Design review of the part built by this model. Coordinates are the model's own, in mm. A direction names the side the tool comes from. Give positions to 0.01 mm unless a question says otherwise; leave off trailing zeros. Order: outer loops, then holes, each group sorted by start corner. A loop starts at its lowest first (then second) coordinate and runs counter-clockwise, first axis right, second up. Notation, with made-up numbers: (-12, 69.25) -> (27, 69.25) arc R18 ccw to (27, 102.25) -> close; hole circle Ø2 at (46.5, -18). An arc over 180 degrees is marked (long way). Return JSON: item names as keys, results as strings.
```python
from build123d import *

# Parameters (mm, degrees)
SKETCH1_R           = 3.75
BOSS_EXTRUDE1_DEPTH = 3.175
SKETCH2_R           = 1.984375
CUT_EXTRUDE1_DEPTH  = 4.175
SKETCH3_W           = 57.15
SKETCH3_H           = 3.175
BOSS_EXTRUDE2_DEPTH = 19.05
SKETCH4_W           = 2.38125
SKETCH4_H           = 2.032
BOSS_EXTRUDE3_DEPTH = 4.7625
SKETCH5_R           = 2.0955
CUT_EXTRUDE2_DEPTH  = 4.175
CHAMFER1_SIZE       = 0.79375
CHAMFER3_SIZE       = 1.5875
FILLET1_R           = 3.175


with BuildPart() as part:
    # Sketch1 → Boss-Extrude1 (new body)
    with BuildSketch(Plane(origin=(0, 0, 0), x_dir=(0, 0, -1), z_dir=(1, 0, 0))):
        with BuildLine():
            Line((-28.575, 0), (28.575, 0))
            Line((28.575, 0), (28.575, 3.175))
            Line((28.575, 3.175), (20.6375, 3.175))
            Line((20.6375, 3.175), (11.1125, 12.7))
            ThreePointArc((11.1125, 12.7), (0, 23.8125), (-11.1125, 12.7))
            Line((-11.1125, 12.7), (-20.6375, 3.175))
            Line((-20.6375, 3.175), (-28.575, 3.175))
            Line((-28.575, 3.175), (-28.575, 0))
        make_face()
        with Locations((0, 12.7)):
            Circle(SKETCH1_R, mode=Mode.SUBTRACT)
    extrude(amount=-BOSS_EXTRUDE1_DEPTH)

    # Sketch2 → Cut-Extrude1 (cut, through all)
    with BuildSketch(Plane(origin=(0, 0, 0), x_dir=(0, 0, -1), z_dir=(1, 0, 0))):
        with Locations((0, 19.812)):
            Circle(SKETCH2_R)
    extrude(amount=-CUT_EXTRUDE1_DEPTH, mode=Mode.SUBTRACT)

    # Sketch3 → Boss-Extrude2 (add)
    with BuildSketch(Plane.ZY.offset(3.175)):
        with Locations((0, 1.5875)):
            Rectangle(SKETCH3_W, SKETCH3_H)
    extrude(amount=BOSS_EXTRUDE2_DEPTH)

    # Sketch4 → Boss-Extrude3 (add)
    with BuildSketch(Plane.ZY.offset(3.175)):
        with Locations((9.128125, 4.191)):
            Rectangle(SKETCH4_W, SKETCH4_H)
    extrude(amount=BOSS_EXTRUDE3_DEPTH)

    # Sketch5 → Cut-Extrude2 (cut, through all)
    with BuildSketch(Plane(origin=(0, 3.175, 0), x_dir=(1, 0, 0), z_dir=(0, 1, 0))):
        with Locations((-11.1125, -19.05)):
            Circle(SKETCH5_R)
        with Locations((-11.1125, 19.05)):
            Circle(SKETCH5_R)
    extrude(amount=-CUT_EXTRUDE2_DEPTH, mode=Mode.SUBTRACT)

    # Chamfer1
    chamfer1_edges = [part.edges().sort_by_distance(p)[0] for p in [
        (-13.208, 3.175, 19.05),
        (-13.208, 3.175, -19.05),
    ]]
    chamfer(chamfer1_edges, length=CHAMFER1_SIZE)

    # Chamfer3
    chamfer3_edges = [part.edges().sort_by_distance(p)[0] for p in [
        (-3.175, 3.175, 15.478125),
        (-3.175, 3.175, -6.35),
    ]]
    chamfer(chamfer3_edges, length=CHAMFER3_SIZE)

    # Fillet1
    fillet1_edges = [part.edges().sort_by_distance(p)[0] for p in [
        (0, 1.5875, -28.575),
        (0, 1.5875, 28.575),
        (-22.225, 1.5875, -28.575),
        (-22.225, 1.5875, 28.575),
    ]]
    fillet(fillet1_edges, radius=FILLET1_R)


solid = part.part
```
Item 1: Add section A-A (x = -5.5). Give the boundary of the cut face in (y, z) (1 decimal).
Result set:
{"outline": "(0, -28.6) -> (3.2, -28.6) -> (3.2, 7.9) -> (5.2, 7.9) -> (5.2, 10.3) -> (3.2, 10.3) -> (3.2, 28.6) -> (0, 28.6) -> close"}
Item 2: For pin 1 (2 mm diameter, centred on x = -6, y = 4.5, fed in from +Z); pin 2 (0.6 mm diameter, centred on x = -6.5, y = 4, fed in from -Z); pin 3 (2.5 mm diameter, centred on x = -6.5, z = 9, fed in from +Y); pin 4 (2.5 mm diameter, centred on y = 19.812, z = 0, fed in from -X), all flat-tipped, find the tip position at first contact; note any pin that passes through.
Result set:
{"pin 1": "stops at z = 10.32", "pin 2": "stops at z = 7.94", "pin 3": "stops at y = 5.21", "pin 4": "passes through"}
Item 3: Add section C-C (x = -11.75). Give the number of separate pieces and of enclosed holes in the cut face, plus the area to 3 significant figures.
Result set:
{"separate pieces": "3", "enclosed holes": "0", "area": "155 mm^2"}
Item 4: Wall thickness on L1, parallel to Y at x = -1, z = 0; L2, parallel to X at y = 0.8, z = -19.05 (3 decimals); L3, parallel to Y at x = -15, z = 20 (3 decimals): over which ranges is each line inside the solid? List them lowest first. Write a range as [from, to].
Result set:
{"L1": "y = [0, 8.95], [16.45, 17.83], [21.8, 23.81]", "L2": "x = [-22.225, -13.208], [-9.017, 0]", "L3": "y = [0, 3.175]"}
Item 5: Mouldability with a two-part tool opening along X and no side actions: class faces 1 (the face through (-1.82, 8, 15.81)), 2 (the face through (-0.955, 1.565, 27.67)), 3 (the face through (-22.225, 2, 0)), 4 (the face through (-10.15, 1.21, -17.19)) as released by +X, released by -X, zero draft, split by the parting line, or undercut.
Result set:
{"face 1": "zero draft", "face 2": "released by +X", "face 3": "released by -X", "face 4": "undercut"}
Item 6: Add section D-D (y = 8.25). Give the boundary of the cut face in (x, z) (1 decimal).
Result set:
{"outline": "(-3.2, -15.6) -> (0, -15.6) -> (0, 15.6) -> (-3.2, 15.6) -> close"}
Item 7: Machinability: for faces 5 (the face through (-1.57, 21.78, 0.26)), 6 (the face through (-3.96, 3.98, 15.41)), 7 (the face through (-7.938, 4, 9)), which of the approach directions +Z, -Z, +X, -X, +Y, -Y give a long, thin tool a straight path to every point of the face, cutting with its end or side? Answer none if there is none.
Result set:
{"face 5": "+X, -X", "face 6": "+Z, -X, +Y", "face 7": "+Z, -Z, -X, +Y"}
Item 8: Add section B-B (z = -9). Give the boundary of the cut face in (x, y) (1 decimal).
Result set:
{"outline": "(-22.2, 0) -> (0, 0) -> (0, 19.2) -> (-3.2, 19.2) -> (-3.2, 4.8) -> (-4.8, 3.2) -> (-22.2, 3.2) -> close"}
